Work out the finished part from the listing and answer in its coordinate system (mm). A direction names the side the tool comes from. Round coordinates to 2 decimals unless told otherwise and drop trailing zeros. Loops run counter-clockwise (first coordinate to the right, second up) from the corner with the lowest first, then second, coordinate; pieces in that order, holes last. Notation, with made-up numbers: (-17, 69.25) -> (15, 69.25) arc R34 ccw to (15, 105.25) -> close; hole circle Ø2 at (-33.5, -8). An arc over 180 degrees is marked (long way). Use one line per item in the form item = value.
```python
from build123d import *

# Parameters (mm, degrees)
F0_R     = 11.3
F0_R_2   = 10.5
F1_DEPTH = 160
F3_DEPTH = 25
F4_COUNT = 3
F4_ANGLE = 30


with BuildPart() as f1:
    # F0 (on Front) → F1 (new body)
    with BuildSketch(Plane.XZ):
        Circle(F0_R)
        Circle(F0_R_2, mode=Mode.SUBTRACT)
    extrude(amount=F1_DEPTH)

    # F2 (on Right) → F3 (join)
    with BuildSketch(Plane.YZ):
        Polygon((-40, 10.536463), (0, 10.536463), (0, 22.977106), (-24.981545, 22.977106), align=None)
    extrude(amount=F3_DEPTH)

    # F4: F1 ×3 about axis
    f4_axis = Axis((0, 0, 0), (0, 1, 0))


with BuildPart() as f1_1:
    add(f1.part)
    for i in range(1, F4_COUNT):
        add(f1.part.rotate(f4_axis, i * F4_ANGLE / (F4_COUNT - 1)))


solid = f1_1.part
```
(1) Find section D-D, the plane x = 17.5. Write down the section's boundary in (y, z), then the cut area to 3 significant figures.
Completed:
outline = (-40, 2.06) -> (0, 2.06) -> (0, 22.98) -> (-24.98, 22.98) -> (-40, 10.54) -> (-34.97, 10.54) -> (-40, 6.22) -> (-35.65, 6.22) -> close
area = 723 mm2
(2) Find section B-B, the plane z = 0. Write down the section's boundary in (x, y), then the cut area to 3 significant figures.
Completed:
outline = (-11.3, -160) -> (-10.5, -160) -> (-10.5, 0) -> (-11.3, 0) -> close; (10.5, -160) -> (11.3, -160) -> (11.3, 0) -> (10.5, 0) -> close; (21.07, -40) -> (28.87, -35.3) -> (28.87, 0) -> (21.07, 0) -> close
area = 549 mm2
(3) For a pull along Z with two mould halves and no side action, classify faces 6 (the flat face through (0, -15, 17)), 7 (the flat face through (12.32, -32.39, 16.84)), 8 (the flat face through (18.88, -37.18, 5.85)) as +Z half, -Z half, draft (parallel to the pull), parting line (faces both ways), or undercut.
Completed:
face_6 = draft
face_7 = +Z half
face_8 = undercut
(4) Find section A-A, the plane y = -15.5. Write down the section's boundary in (x, z).
Completed:
outline = (0, 11.3) arc R11.3 ccw (long way) to (8.8, 7.08) -> (26.92, -3.38) -> (33.14, 7.4) -> (28.57, 10.04) -> (30.1, 15.72) -> (25, 17.09) -> (25, 22.98) -> (0, 22.98) -> close; hole circle Ø21 at (0, 0)
(5) Find section C-C, the plane z = -7. Write down the section's boundary in (x, y).
Completed:
outline = (-8.87, -160) -> (-7.83, -160) -> (-7.83, 0) -> (-8.87, 0) -> close; (7.83, -160) -> (8.87, -160) -> (8.87, 0) -> (7.83, 0) -> close
(6) For faces 1 (the flat face through (30.82, -12.32, 8.74)), 2 (the flat face through (25, -20, 18)), 3 (the flat face through (30.073, -15.836, 2.087)), 4 (the flat face through (27.512, -12.316, 16.416)), 5 (the flat face through (28.865, -20.28, 11.135)), determine the directions among +Z, -Z, +X, -X, +Y, -Y from which every point of the face is accessible in a straight line to the end or side of a thin tool.
Completed:
face_1 = +X, +Y, -Y
face_2 = +Z, +X, -Y
face_3 = -Z, +X, +Y, -Y
face_4 = +Z, +X, +Y, -Y
face_5 = +X, -Y
(7) Given P1, Ø8, axis at x = -4, y = -79, coming from the +Z side; P2, Ø12, axis at y = -43.5, z = 8, coming from the -X side; P3, Ø10, axis at y = -80.5, z = 18.5, coming from the +X side; P4, Ø13.5, axis at y = -27.5, z = 17.5, coming from the +X side, each flat-ended and moving along its own axis, determine where each tip first touches the part or whether it passes through.
Completed:
P1 = 11.3
P2 = -11.12
P3 = through
P4 = 30.1
(8) Consider L1, parallel to Z at x = 0, y = -54; L2, parallel to X at y = -108, z = 0.5; L3, parallel to X at y = -81, z = 5. Determine where each line is inside the solid, lowest interval first.
Completed:
L1 = -11.3 to -10.5, 10.5 to 11.3
L2 = -11.29 to -10.49, 10.49 to 11.29
L3 = -10.13 to -9.23, 9.23 to 10.13
